from build123d import *

# Parameters (mm, degrees)
ESQUISSE1_R             = 14
BOSS_EXTRU_1_DEPTH      = 13
BOSS_EXTRU_2_START      = -2
ESQUISSE3_R             = 14
BOSS_EXTRU_2_DEPTH      = 2
ESQUISSE4_W             = 13
ESQUISSE4_H             = 10.015892944
ENL_V_MAT_EXTRU_1_DEPTH = 60


with BuildPart() as part:
    # Esquisse1 → Boss.-Extru.1 (new body)
    with BuildSketch(Plane.XY):
        with BuildLine():
            ThreePointArc((-25, 0), (0, 25), (25, 0))
            Line((25, 0), (25, -32.475372295))
            Line((25, -32.475372295), (-25, -32.475372295))
            Line((-25, -32.475372295), (-25, 0))
        make_face()
        with Locations(Location((0, 0, 0), (0, 0, 180))):
            Circle(ESQUISSE1_R, mode=Mode.SUBTRACT)
    extrude(amount=BOSS_EXTRU_1_DEPTH)

    # Esquisse3 → Boss.-Extru.2 (add)
    with BuildSketch(Plane.XY.offset(13).offset(BOSS_EXTRU_2_START)):
        with Locations(Location((0, 0, 0), (0, 0, 180))):
            Circle(ESQUISSE3_R)
    extrude(amount=BOSS_EXTRU_2_DEPTH)

    # Esquisse4 → Enlèv. mat.-Extru.1 (cut)
    with BuildSketch(Plane.ZY.offset(25)):
        with Locations((6.5, -29.313318767)):
            Rectangle(ESQUISSE4_W, ESQUISSE4_H)
    extrude(amount=-ENL_V_MAT_EXTRU_1_DEPTH, mode=Mode.SUBTRACT)


solid = part.part
For this review, take the finished solid that the model builds, in its own axes (mm). Round coordinates to 2 decimals unless told otherwise and drop trailing zeros. Write each loop counter-clockwise with the first axis right and the second up, starting at its lowest first coordinate (ties: lowest second). Pieces come first, ordered by that corner, then holes. Notation, with made-up numbers: (15.25, 38) -> (33.25, 38) arc R25 ccw to (33.25, 57) -> close; hole circle Ø6 at (-23.5, 57). An arc over 180 degrees is marked (long way). Use CSV: the item, a comma, the result in double quotes.
(1) Consider section C-C, the plane y = -11.5. Give the boundary of the cut face in (x, z).
Computed values:
outline,"(-25, 0) -> (-7.98, 0) -> (-7.98, 11) -> (7.98, 11) -> (7.98, 0) -> (25, 0) -> (25, 13) -> (-25, 13) -> close"
(2) Consider section D-D, the plane z = 12. Give the boundary of the cut face in (x, y), plus the area to 3 significant figures.
Computed values:
outline,"(-25, -24.31) -> (25, -24.31) -> (25, 0) arc R25 ccw to (-25, 0) -> close"
area,"2,200 mm²"
(3) Consider section B-B, the plane x = 0. Give the boundary of the cut face in (y, z).
Computed values:
outline,"(-24.31, 0) -> (-14, 0) -> (-14, 11) -> (14, 11) -> (14, 0) -> (25, 0) -> (25, 13) -> (-24.31, 13) -> close"
(4) Consider section A-A, the plane z = 5.5. Give the boundary of the cut face in (x, y), plus the area to 3 significant figures.
Computed values:
outline,"(-25, -24.31) -> (25, -24.31) -> (25, 0) arc R25 ccw to (-25, 0) -> close; hole circle Ø28 at (0, 0)"
area,"1,580 mm²"
(5) Clearance check with flat-ended pins moving along their axes: P1, Ø5, axis at x = -3.5, y = 4.5, coming from the -Z side; P2, Ø3, axis at y = 3, z = 2.5, coming from the +X side. State where each tip first meets the part, or that it passes through.
Computed values:
P1,"z = 11"
P2,"x = 24.95"
(6) Draft analysis for pull direction Y (two halves, no side actions). For faces 1 (the face through (-25, -12, 6)), 2 (the face through (-12.932, 5.362, 5.423)), 3 (the face through (0, 0, 11)), 4 (the face through (0, -24.305, 6)), state which applies: +Y half, -Y half, draft (parallel to the pull), parting line (faces both ways), or undercut.
Computed values:
face 1,"draft"
face 2,"undercut"
face 3,"undercut"
face 4,"-Y half"
(7) To check wall thickness, follow L1, parallel to Y at x = 0, z = 8.25; L2, parallel to Z at x = -1.5, y = -12.5; L3, parallel to X at y = -3.5, z = 9. State the ranges of each line that lie inside material, in increasing order. Write a range as [from, to].
Computed values:
L1,"[-24.31, -14], [14, 25]"
L2,"[11, 13]"
L3,"[-25, -13.56], [13.56, 25]"
